from build123d import *

# Parameters (mm, degrees)
F0_R     = 2.474548
F1_DEPTH = 0.25
F2_DEPTH = 0.25
F3_R     = 2.476563
F4_DEPTH = 0.25


with BuildPart() as f1:
    # F0 (on Top) → F1 (new body)
    with BuildSketch(Plane.XY):
        with BuildLine():
            Line((8.609738, -2.39951), (8.609738, 2.438852))
            ThreePointArc((8.609738, 2.438852), (2.404608, 0.019671), (8.609738, -2.39951))
        make_face()
        with Locations((5.978753, 0.019671)):
            Circle(F0_R, mode=Mode.SUBTRACT)
        with Locations((5.978753, 0.019671)):
            Circle(F0_R)
        with BuildLine():
            ThreePointArc((8.609738, -2.39951), (9.308771, -1.278596), (9.552899, 0.019671))
            ThreePointArc((9.552899, 0.019671), (9.308771, 1.317938), (8.609738, 2.438852))
            Line((8.609738, 2.438852), (8.609738, -2.39951))
        make_face()
    extrude(amount=F1_DEPTH)

    # F0 (on Top) → F2 (join)
    with BuildSketch(Plane.XY):
        with BuildLine():
            ThreePointArc((8.609738, 2.438852), (9.308771, 1.317938), (9.552899, 0.019671))
            ThreePointArc((9.552899, 0.019671), (9.308771, -1.278596), (8.609738, -2.39951))
            Line((8.609738, -2.39951), (8.609738, -3.555269))
            Line((8.609738, -3.555269), (9.709738, -3.555269))
            Line((9.709738, -3.555269), (9.709738, 3.593735))
            Line((9.709738, 3.593735), (8.609738, 3.593735))
            Line((8.609738, 3.593735), (8.609738, 2.438852))
        make_face()
    extrude(amount=F2_DEPTH)

    # F3 (on face) → F4 (cut)
    with BuildSketch(Plane.XY.offset(0.25)):
        with Locations((5.978753, 0.019671)):
            Circle(F3_R)
    extrude(amount=-F4_DEPTH, mode=Mode.SUBTRACT)


solid = f1.part
CAD build for the part. Positions are in the model's coordinates, mm. Coordinates: 2 decimals unless noted, no trailing zeros. Loops run counter-clockwise (first coordinate to the right, second up) from the corner with the lowest first, then second, coordinate; pieces in that order, holes last. Notation, with made-up numbers: (77.5, 66) - (92.5, 66) arc R27 ccw to (92.5, 92) - close; hole circle Ø11 at (40.25, -28.5). An arc over 180 degrees is marked (long way). Use one line per item in the form item = value. Start each with the question number.
1) Band-saw the part on A-A (y = -1.75). Give the cut face in (x, z), and give its area (3 significant figures).
2) Band-saw the part on D-D (x = 3). Give the cut face in (y, z), and give its area (3 significant figures).
3) Drill centre lines: L1, parallel to Y at x = 6, z = 0.1; L2, parallel to X at y = -3.25, z = 0.2; L3, parallel to Y at x = 6.75, z = 0.1. Where is each one in solid material? Low to high. Write a range as from..to.
4) Band-saw the part on C-C (z = 0.1). Give the cut face in (x, y), and give its area (3 significant figures).
5) Band-saw the part on B-B (x = 7.25). Give the cut face in (y, z).
Check values:
q1.outline = (2.87, 0) - (4.25, 0) - (4.25, 0.25) - (2.87, 0.25) - close; (7.71, 0) - (9.71, 0) - (9.71, 0.25) - (7.71, 0.25) - close
q1.area = 0.843 mm2
q2.outline = (-1.96, 0) - (1.99, 0) - (1.99, 0.25) - (-1.96, 0.25) - close
q2.area = 0.988 mm2
q3.L1 = -3.55..-2.46, 2.5..3.59
q3.L2 = 4.54..7.42, 8.61..9.71
q3.L3 = -3.47..-2.33, 2.37..3.51
q4.outline = (8.61, -3.56) - (9.71, -3.56) - (9.71, 3.59) - (8.61, 3.59) - (8.61, 2.44) arc R3.57 ccw (long way) to (8.61, -2.4) - close; hole circle Ø4.95 at (5.98, 0.02)
q4.area = 25.6 mm2
q5.outline = (-3.32, 0) - (-2.11, 0) - (-2.11, 0.25) - (-3.32, 0.25) - close; (2.15, 0) - (3.36, 0) - (3.36, 0.25) - (2.15, 0.25) - close
